```python
from build123d import *

# Parameters (mm, degrees)
SKETCH2_R           = 5
BOSS_EXTRUDE1_DEPTH = 5


with BuildPart() as part:
    # Sketch2 → Boss-Extrude1 (new, symmetric)
    with BuildSketch(Plane(origin=(0, 0, 0), x_dir=(1, 0, 0), z_dir=(0, 1, 0))):
        with BuildLine():
            Line((107.901994577, 25), (147.901994577, 25))
            ThreePointArc((147.901994577, 25), (106.066017178, 106.066017178), (25, 147.901994577))
            Line((25, 147.901994577), (25, 107.901994577))
            Line((25, 107.901994577), (-25, 107.901994577))
            Line((-25, 107.901994577), (-25, 147.901994577))
            ThreePointArc((-25, 147.901994577), (-106.066017178, 106.066017178), (-147.901994577, 25))
            Line((-147.901994577, 25), (-107.901994577, 25))
            Line((-107.901994577, 25), (-107.901994577, -25))
            Line((-107.901994577, -25), (-147.901994577, -25))
            ThreePointArc((-147.901994577, -25), (-106.066017178, -106.066017178), (-25, -147.901994577))
            Line((-25, -147.901994577), (-25, -107.901994577))
            Line((-25, -107.901994577), (25, -107.901994577))
            Line((25, -107.901994577), (25, -147.901994577))
            ThreePointArc((25, -147.901994577), (106.066017178, -106.066017178), (147.901994577, -25))
            Line((147.901994577, -25), (107.901994577, -25))
            Line((107.901994577, -25), (107.901994577, 25))
        make_face()
        with Locations(Location((0, 0, 0), (0, 0, 270))):
            Circle(SKETCH2_R, mode=Mode.SUBTRACT)
    extrude(amount=BOSS_EXTRUDE1_DEPTH, both=True)


solid = part.part
```
Source: CAD feature listing. Evaluate the final solid. Frame: model axes, mm. A direction names the side the tool comes from. Round coordinates to 2 decimals unless told otherwise and drop trailing zeros. Order: outer loops, then holes, each group sorted by start corner. A loop starts at its lowest first (then second) coordinate and runs counter-clockwise, first axis right, second up. Notation, with made-up numbers: (40, 75.5) -> (83, 75.5) arc R16 cw to (83, 93.5) -> close; hole circle Ø6 at (81.5, 55.25). An arc over 180 degrees is marked (long way). One line per item, written item: value. Start each with the question number.
Q1. Material intervals for probe 1 along X at (y, z) = (-2.25, 0); probe 2 along X at (y, z) = (3.25, -10); probe 3 along Z at (x, y) = (-110, -1.25), sorted ascending.
Q2. Section query A-A (z = 0). Return the cut outline in (x, y).
Q3. Draft query along Z for faces 4 (the flat face through (0, 0, 107.902)), 5 (the flat face through (128, 0, 25)), 6 (the flat face through (0, 0, -107.902)), 7 (the flat face through (25, 0, -128)). Return one class per face: pulls with the +Z half, pulls with the -Z half, needs draft (parallel to the pull), parting line crosses it, or undercut.
Q4. Access query for faces 1 (the flat face through (128, 0, -25)), 2 (the flat face through (-25, 0, 128)), 3 (the flat face through (-128, 0, 25)). Directions: +Z, -Z, +X, -X, +Y, -Y. A direction counts if a zero-diameter tool reaches every point of the face in a straight line with its end or side. Return the directions, or none.
Q5. Section query C-C (x = 0). Return the cut outline in (y, z).
Q6. Pin query (flat end, axial travel): pin 1 (5 mm diameter, centred on x = 130.5, y = 1.5, fed in from -Z); pin 2 (1.5 mm diameter, centred on x = -2.5, y = 4, fed in from +Z); pin 3 (3 mm diameter, centred on y = -2.5, z = -133, fed in from -X). Return the tip coordinate at first contact, or that it passes through.
Q7. Section query B-B (y = 1.5). Return the cut outline in (x, z), plus the area to 3 significant figures.
Q8. Section query D-D (z = -55.5). Return the cut outline in (x, y), plus the area to 3 significant figures.
Findings below:
1. probe 1: -107.9 to -5, 5 to 107.9
1. probe 2: -107.9 to 107.9
1. probe 3: -101.98 to -25, 25 to 101.98
2. outline: (-107.9, -5) -> (-5, -5) -> (-5, 5) -> (-107.9, 5) -> close; (5, -5) -> (107.9, -5) -> (107.9, 5) -> (5, 5) -> close
3. face 4: pulls with the +Z half
3. face 5: undercut
3. face 6: pulls with the -Z half
3. face 7: needs draft
4. face 1: +X, +Y, -Y
4. face 2: +Z, +Y, -Y
4. face 3: -X, +Y, -Y
5. outline: (-5, -107.9) -> (5, -107.9) -> (5, -5) -> (-5, -5) -> close; (-5, 5) -> (5, 5) -> (5, 107.9) -> (-5, 107.9) -> close
6. pin 1: z = -78.2
6. pin 2: z = 107.9
6. pin 3: x = -72.16
7. outline: (-147.9, -25) arc R150 ccw to (-25, -147.9) -> (-25, -107.9) -> (25, -107.9) -> (25, -147.9) arc R150 ccw to (147.9, -25) -> (107.9, -25) -> (107.9, 25) -> (147.9, 25) arc R150 ccw to (25, 147.9) -> (25, 107.9) -> (-25, 107.9) -> (-25, 147.9) arc R150 ccw to (-147.9, 25) -> (-107.9, 25) -> (-107.9, -25) -> close; hole circle Ø10 at (0, 0)
7. area: 62,300 mm²
8. outline: (-139.35, -5) -> (139.35, -5) -> (139.35, 5) -> (-139.35, 5) -> close
8. area: 2,790 mm²
